For this review, take the finished solid that the model builds, in its own axes (mm). A direction names the side the tool comes from. Give positions to 0.01 mm unless a question says otherwise; leave off trailing zeros. Order: outer loops, then holes, each group sorted by start corner. A loop starts at its lowest first (then second) coordinate and runs counter-clockwise, first axis right, second up.
Item 1: Machinability: for faces 1 (the flat face through (6, 8, 4)), 2 (the flat face through (19, 14, 3.3)), 3 (the flat face through (69, 2.25, 6)), which of the approach directions +Z, -Z, +X, -X, +Y, -Y give a long, thin tool a straight path to every point of the face, cutting with its end or side? Answer none if there is none.
Item 2: Consider section C-C (x = 47.5). Give the boundary of the cut face in (y, z), plus the area to 3 significant figures.
Item 3: Consider section B-B (z = -71). Give the boundary of the cut face in (x, y), plus the area to 3 significant figures.
Item 4: Consider section A-A (y = 14). Give the boundary of the cut face in (x, z).
Item 5: Consider section D-D (z = -27). Give the boundary of the cut face in (x, y), plus the area to 3 significant figures.
Item 6: For probe 1 along X at (y, z) = (1.25, -27); probe 2 along X at (y, z) = (1.2, -4); probe 3 along Z at (x, y) = (119.5, 0.75), list the stretches that pass through material, from the lowest coordinate up.
Item 7: For P1, Ø3, axis at x = 22.5, z = -43, coming from the -Y side; P2, Ø2.5, axis at x = 58.5, y = 5.5, coming from the -Z side; P3, Ø2, axis at y = 7, z = 2, coming from the +X side; P4, Ø12, axis at x = 70.5, z = -40.5, coming from the -Y side, all flat-tipped, find the tip position at first contact; note any pin that passes through.
Item 8: The part is to be moulded in two halves that separate along Z. For faces 4 (the cylindrical face through (23.58, 1.11, -28.18)), 5 (the flat face through (19, 10.75, -3)), 6 (the flat face through (69, 10, 12.8)), 7 (the cylindrical face through (3.57, 1.11, -5.6)), say which applies: released by +Z, released by -Z, zero draft, split by the parting line, or undercut.
```python
from build123d import *

# Parameters (mm, degrees)
SKETCH1_W           = 123
SKETCH1_H           = 75
SKETCH1_R           = 1.6
BOSS_EXTRUDE1_DEPTH = 2.25
SKETCH2_W           = 25.5
SKETCH2_H           = 22
SKETCH2_W_2         = 61
BOSS_EXTRUDE2_DEPTH = 8.5
SKETCH3_W           = 25.5
SKETCH3_H           = 9.5
SKETCH3_W_2         = 61
BOSS_EXTRUDE3_DEPTH = 7


with BuildPart() as part:
    # Sketch1 → Boss-Extrude1 (new body)
    with BuildSketch(Plane(origin=(0, 0, 0), x_dir=(1, 0, 0), z_dir=(0, 1, 0))):
        with Locations((61.5, 37.5)):
            Rectangle(SKETCH1_W, SKETCH1_H)
        with Locations(Location((119.5, 71, 0), (0, 0, 270))):
            Circle(SKETCH1_R, mode=Mode.SUBTRACT)
        with Locations(Location((119.5, 4, 0), (0, 0, 270))):
            Circle(SKETCH1_R, mode=Mode.SUBTRACT)
        with Locations(Location((3.5, 4, 0), (0, 0, 270))):
            Circle(SKETCH1_R, mode=Mode.SUBTRACT)
        with Locations(Location((22.5, 43, 0), (0, 0, 270))):
            Circle(SKETCH1_R, mode=Mode.SUBTRACT)
        with Locations(Location((47.5, 43, 0), (0, 0, 270))):
            Circle(SKETCH1_R, mode=Mode.SUBTRACT)
        with Locations(Location((22.5, 27, 0), (0, 0, 270))):
            Circle(SKETCH1_R, mode=Mode.SUBTRACT)
        with Locations(Location((47.5, 27, 0), (0, 0, 270))):
            Circle(SKETCH1_R, mode=Mode.SUBTRACT)
    extrude(amount=BOSS_EXTRUDE1_DEPTH)

    # Sketch2 → Boss-Extrude2 (add)
    with BuildSketch(Plane(origin=(0, 2.25, 0), x_dir=(1, 0, 0), z_dir=(0, 1, 0))):
        with Locations((18.75, -1.8)):
            Rectangle(SKETCH2_W, SKETCH2_H)
        with Locations((69.5, -1.8)):
            Rectangle(SKETCH2_W_2, SKETCH2_H)
    extrude(amount=BOSS_EXTRUDE2_DEPTH)

    # Sketch3 → Boss-Extrude3 (add)
    with BuildSketch(Plane(origin=(0, 10.75, 0), x_dir=(1, 0, 0), z_dir=(0, 1, 0))):
        with Locations((18.75, -8.05)):
            Rectangle(SKETCH3_W, SKETCH3_H)
        with Locations((69.5, -8.05)):
            Rectangle(SKETCH3_W_2, SKETCH3_H)
    extrude(amount=BOSS_EXTRUDE3_DEPTH)


solid = part.part
```
Resolved:
1. face 1: +Z, -Z, -X, +Y
1. face 2: -Z, +X, -X, +Y
1. face 3: +Z, +X, -X, -Y
2. outline: (0, -75) - (2.25, -75) - (2.25, -44.6) - (0, -44.6) - close; (0, -41.4) - (2.25, -41.4) - (2.25, -28.6) - (0, -28.6) - close; (0, -25.4) - (2.25, -25.4) - (2.25, -9.2) - (10.75, -9.2) - (10.75, 3.3) - (17.75, 3.3) - (17.75, 12.8) - (2.25, 12.8) - (2.25, 0) - (0, 0) - close
2. area: 408 mm2
3. outline: (0, 0) - (117.9, 0) - (117.9, 2.25) - (0, 2.25) - close; (121.1, 0) - (123, 0) - (123, 2.25) - (121.1, 2.25) - close
3. area: 270 mm2
4. outline: (6, 3.3) - (31.5, 3.3) - (31.5, 12.8) - (6, 12.8) - close; (39, 3.3) - (100, 3.3) - (100, 12.8) - (39, 12.8) - close
5. outline: (0, 0) - (20.9, 0) - (20.9, 2.25) - (0, 2.25) - close; (24.1, 0) - (45.9, 0) - (45.9, 2.25) - (24.1, 2.25) - close; (49.1, 0) - (123, 0) - (123, 2.25) - (49.1, 2.25) - close
5. area: 262 mm2
6. probe 1: x = 0 to 20.9, 24.1 to 45.9, 49.1 to 123
6. probe 2: x = 0 to 1.9, 5.1 to 117.9, 121.1 to 123
6. probe 3: z = -75 to -72.6, -69.4 to -5.6, -2.4 to 0
7. P1: passes through
7. P2: stops at z = -9.2
7. P3: stops at x = 100
7. P4: stops at y = 0
8. face 4: undercut
8. face 5: zero draft
8. face 6: released by +Z
8. face 7: undercut
